Geometry: final body of the model. Coordinates: model frame, mm. A direction names the side the tool comes from. Give positions to 0.01 mm unless a question says otherwise; leave off trailing zeros. Loops run counter-clockwise (first coordinate to the right, second up) from the corner with the lowest first, then second, coordinate; pieces in that order, holes last. Notation, with made-up numbers: (-28, 37) - (-9, 37) arc R28 ccw to (-9, 75) - close; hole circle Ø6 at (21, 33.5). An arc over 180 degrees is marked (long way). Answer in a Markdown table with one row per item.
from build123d import *

# Parameters (mm, degrees)
CROQUIS2_W              = 80
CROQUIS2_H              = 45
SALIENTE_EXTRUIR1_DEPTH = 8
CORTAR_EXTRUIR1_DEPTH   = 3
CROQUIS4_W              = 5
CROQUIS4_H              = 15
SALIENTE_EXTRUIR2_DEPTH = 35
CORTAR_EXTRUIR2_DEPTH   = 34.5
REDONDEO1_R             = 5
CROQUIS6_W              = 10
CROQUIS6_H              = 5.6
CORTAR_EXTRUIR3_DEPTH   = 3
CROQUIS8_W              = 15
CROQUIS8_H              = 8
CORTAR_EXTRUIR4_DEPTH   = 34.5
REDONDEO2_R             = 2


with BuildPart() as part:
    # Croquis2 → Saliente-Extruir1 (new body)
    with BuildSketch(Plane(origin=(0, 0, 0), x_dir=(1, 0, 0), z_dir=(0, 1, 0))):
        Rectangle(CROQUIS2_W, CROQUIS2_H)
        with BuildLine():
            Line((-20.5, 14.6), (-14.5, 14.6))
            ThreePointArc((-14.5, 14.6), (-12.9, 13), (-14.5, 11.4))
            Line((-14.5, 11.4), (-20.5, 11.4))
            ThreePointArc((-20.5, 11.4), (-22.1, 13), (-20.5, 14.6))
        make_face(mode=Mode.SUBTRACT)
        with BuildLine():
            Line((20.5, 14.6), (14.5, 14.6))
            ThreePointArc((14.5, 14.6), (12.9, 13), (14.5, 11.4))
            Line((14.5, 11.4), (20.5, 11.4))
            ThreePointArc((20.5, 11.4), (22.1, 13), (20.5, 14.6))
        make_face(mode=Mode.SUBTRACT)
        with BuildLine():
            Line((20.5, -14.6), (14.5, -14.6))
            ThreePointArc((14.5, -14.6), (12.9, -13), (14.5, -11.4))
            Line((14.5, -11.4), (20.5, -11.4))
            ThreePointArc((20.5, -11.4), (22.1, -13), (20.5, -14.6))
        make_face(mode=Mode.SUBTRACT)
        with BuildLine():
            Line((-20.5, -14.6), (-14.5, -14.6))
            ThreePointArc((-14.5, -14.6), (-12.9, -13), (-14.5, -11.4))
            Line((-14.5, -11.4), (-20.5, -11.4))
            ThreePointArc((-20.5, -11.4), (-22.1, -13), (-20.5, -14.6))
        make_face(mode=Mode.SUBTRACT)
        with BuildLine():
            Line((-20.5, 1.6), (-14.5, 1.6))
            ThreePointArc((-14.5, 1.6), (-12.9, 0), (-14.5, -1.6))
            Line((-14.5, -1.6), (-20.5, -1.6))
            ThreePointArc((-20.5, -1.6), (-22.1, 0), (-20.5, 1.6))
        make_face(mode=Mode.SUBTRACT)
        with BuildLine():
            Line((20.5, 1.6), (14.5, 1.6))
            ThreePointArc((14.5, 1.6), (12.9, 0), (14.5, -1.6))
            Line((14.5, -1.6), (20.5, -1.6))
            ThreePointArc((20.5, -1.6), (22.1, 0), (20.5, 1.6))
        make_face(mode=Mode.SUBTRACT)
        with BuildLine():
            Line((-3, 14.6), (3, 14.6))
            ThreePointArc((3, 14.6), (4.6, 13), (3, 11.4))
            Line((3, 11.4), (-3, 11.4))
            ThreePointArc((-3, 11.4), (-4.6, 13), (-3, 14.6))
        make_face(mode=Mode.SUBTRACT)
        with BuildLine():
            Line((-3, -11.4), (3, -11.4))
            ThreePointArc((3, -11.4), (4.6, -13), (3, -14.6))
            Line((3, -14.6), (-3, -14.6))
            ThreePointArc((-3, -14.6), (-4.6, -13), (-3, -11.4))
        make_face(mode=Mode.SUBTRACT)
    extrude(amount=SALIENTE_EXTRUIR1_DEPTH)

    # Croquis3 → Cortar-Extruir1 (cut)
    with BuildSketch(Plane(origin=(0, 8, 0), x_dir=(1, 0, 0), z_dir=(0, 1, 0))):
        with BuildLine():
            Line((-20.5, 16), (-14.5, 16))
            ThreePointArc((-14.5, 16), (-11.5, 13), (-14.5, 10))
            Line((-14.5, 10), (-20.5, 10))
            ThreePointArc((-20.5, 10), (-23.5, 13), (-20.5, 16))
        make_face()
        with BuildLine():
            Line((20.5, 16), (14.5, 16))
            ThreePointArc((14.5, 16), (11.5, 13), (14.5, 10))
            Line((14.5, 10), (20.5, 10))
            ThreePointArc((20.5, 10), (23.5, 13), (20.5, 16))
        make_face()
        with BuildLine():
            Line((20.5, -16), (14.5, -16))
            ThreePointArc((14.5, -16), (11.5, -13), (14.5, -10))
            Line((14.5, -10), (20.5, -10))
            ThreePointArc((20.5, -10), (23.5, -13), (20.5, -16))
        make_face()
        with BuildLine():
            Line((-20.5, -16), (-14.5, -16))
            ThreePointArc((-14.5, -16), (-11.5, -13), (-14.5, -10))
            Line((-14.5, -10), (-20.5, -10))
            ThreePointArc((-20.5, -10), (-23.5, -13), (-20.5, -16))
        make_face()
    extrude(amount=-CORTAR_EXTRUIR1_DEPTH, mode=Mode.SUBTRACT)

    # Croquis4 → Saliente-Extruir2 (add)
    with BuildSketch(Plane.XZ):
        with Locations((9, 0)):
            Rectangle(CROQUIS4_W, CROQUIS4_H)
    extrude(amount=SALIENTE_EXTRUIR2_DEPTH)

    # Croquis5 → Cortar-Extruir2 (cut, through all)
    with BuildSketch(Plane.ZY.offset(-6.5)):
        with BuildLine():
            Line((1.6, -11.25), (1.6, -13.75))
            ThreePointArc((1.6, -13.75), (0, -15.35), (-1.6, -13.75))
            Line((-1.6, -13.75), (-1.6, -11.25))
            ThreePointArc((-1.6, -11.25), (0, -9.65), (1.6, -11.25))
        make_face()
        with BuildLine():
            Line((1.6, -23.75), (1.6, -21.25))
            ThreePointArc((1.6, -21.25), (0, -19.65), (-1.6, -21.25))
            Line((-1.6, -21.25), (-1.6, -23.75))
            ThreePointArc((-1.6, -23.75), (0, -25.35), (1.6, -23.75))
        make_face()
    extrude(amount=-CORTAR_EXTRUIR2_DEPTH, mode=Mode.SUBTRACT)

    # Redondeo1
    redondeo1_edges = [part.edges().sort_by_distance(p)[0] for p in [
        (9, 0, 7.5),
        (9, 0, -7.5),
    ]]
    fillet(redondeo1_edges, radius=REDONDEO1_R)

    # Croquis6 → Cortar-Extruir3 (cut)
    with BuildSketch(Plane.XZ):
        with Locations((-17.5, 0)):
            Rectangle(CROQUIS6_W, CROQUIS6_H)
        with Locations((17.5, 0)):
            Rectangle(CROQUIS6_W, CROQUIS6_H)
        with Locations((0, 13)):
            Rectangle(CROQUIS6_W, CROQUIS6_H)
        with Locations((0, -13)):
            Rectangle(CROQUIS6_W, CROQUIS6_H)
    extrude(amount=-CORTAR_EXTRUIR3_DEPTH, mode=Mode.SUBTRACT)

    # Croquis8 → Cortar-Extruir4 (cut, through all)
    with BuildSketch(Plane.ZY.offset(-6.5)):
        with Locations((0, -31)):
            Rectangle(CROQUIS8_W, CROQUIS8_H)
    extrude(amount=-CORTAR_EXTRUIR4_DEPTH, mode=Mode.SUBTRACT)

    # Redondeo2
    redondeo2_edges = [part.edges().sort_by_distance(p)[0] for p in [
        (9, -27, -7.5),
        (9, -27, 7.5),
        (40, 4, 22.5),
        (-40, 4, 22.5),
        (-40, 4, -22.5),
        (40, 4, -22.5),
    ]]
    fillet(redondeo2_edges, radius=REDONDEO2_R)


solid = part.part
Q1. Cut plane A-A (x = 7.5). Output: boundary loops of the cut face in (y, z).
Check values:
| item | result |
|---|---|
| outline | (-27, -5.5) arc R2 ccw to (-25, -7.5) - (-5, -7.5) arc R5 cw to (0, -12.5) - (0, -22.5) - (8, -22.5) - (8, 22.5) - (0, 22.5) - (0, 12.5) arc R5 cw to (-5, 7.5) - (-25, 7.5) arc R2 ccw to (-27, 5.5) - close; hole (-23.75, -1.6) - (-21.25, -1.6) arc R1.6 ccw to (-21.25, 1.6) - (-23.75, 1.6) arc R1.6 ccw to start; hole (-13.75, -1.6) - (-11.25, -1.6) arc R1.6 ccw to (-11.25, 1.6) - (-13.75, 1.6) arc R1.6 ccw to start |
Q2. Draft query along X for faces 1 (the flat face through (9, -23, 1.6)), 2 (the flat face through (-17, 7, 10)), 3 (the flat face through (11.5, -13, -3)). Return one class per face: pulls with the +X half, pulls with the -X half, needs draft (parallel to the pull), parting line crosses it, or undercut.
Check values:
| item | result |
|---|---|
| face 1 | needs draft |
| face 2 | undercut |
| face 3 | pulls with the +X half |
Q3. Reachability of faces 4 (the flat face through (-12.5, 1, 0)), 5 (the cylindrical face through (11.5, 6.5, -13.1)), 6 (the flat face through (0, 5, -11.4)), 7 (the cylindrical face through (8.96, -25.35, -0.04)) from +Z, -Z, +X, -X, +Y, -Y: full face, straight path, thin tool, end or side. Return the list, or none.
Check values:
| item | result |
|---|---|
| face 4 | -Y |
| face 5 | +Y |
| face 6 | +Y, -Y |
| face 7 | +X, -X |
Q4. Cut plane D-D (y = -3.5). Output: boundary loops of the cut face in (x, z).
Check values:
| item | result |
|---|---|
| outline | (6.5, -7.73) - (11.5, -7.73) - (11.5, 7.73) - (6.5, 7.73) - close |
Q5. Material intervals for line 1 along Z through (x, y) = (8, -12); line 2 along X through (y, z) = (6, -1); line 3 along X through (y, z) = (-6, -2.5), sorted ascending.
Check values:
| item | result |
|---|---|
| line 1 | -7.5 to -1.6, 1.6 to 7.5 |
| line 2 | -40 to -21.75, -13.25 to 13.25, 21.75 to 40 |
| line 3 | 6.5 to 11.5 |
Q6. Cut plane C-C (x = 35). Output: boundary loops of the cut face in (y, z), and give its area (3 significant figures).
Check values:
| item | result |
|---|---|
| outline | (0, -22.5) - (8, -22.5) - (8, 22.5) - (0, 22.5) - close |
| area | 360 mm² |
Q7. First-contact query: pin 1 (8 mm diameter, centred on x = 13, z = -1.5, fed in from -Y); pin 2 (7.5 mm diameter, centred on y = -12.5, z = 5.5, fed in from +X); pin 3 (0.8 mm diameter, centred on x = 8.5, y = -13, fed in from -Z); pin 4 (1 mm diameter, centred on x = -2.5, z = 4, fed in from -Y). Flat tips, straight axial feed; report the tip coordinate or a pass-through.
Check values:
| item | result |
|---|---|
| pin 1 | y = -27 |
| pin 2 | x = 11.5 |
| pin 3 | z = -7.5 |
| pin 4 | y = 0 |
Q8. Cut plane B-B (z = 0). Give the number of separate pieces and of enclosed holes in the cut face, and give its area (3 significant figures).
Check values:
| item | result |
|---|---|
| separate pieces | 5 |
| enclosed holes | 0 |
| area | 566 mm² |
